Source: CAD feature listing. Evaluate the final solid. Frame: model axes, mm. A direction names the side the tool comes from. Give positions to 0.01 mm unless a question says otherwise; leave off trailing zeros. Loops run counter-clockwise (first coordinate to the right, second up) from the corner with the lowest first, then second, coordinate; pieces in that order, holes last. Notation, with made-up numbers: M 31,53.25 L 75,53.25 A21 cw 75,64.25 Z; hole C -6.5,0 d2. An arc over 180 degrees is marked long. Put each result on its own line as item: value.
from build123d import *

# Parameters (mm, degrees)
F0_R      = 37.95
F1_DEPTH  = 5
F2_R      = 36.45
F3_DEPTH  = 5
F4_R      = 3.25
F5_DEPTH  = 10
F6_R      = 12.5
F7_DEPTH  = 25
F8_R      = 9
F9_DEPTH  = 25
F10_R     = 1.5
F11_DEPTH = 10
F12_R     = 1.5
F13_DEPTH = 10


with BuildPart() as f1:
    # F0 (on Top) → F1 (new body)
    with BuildSketch(Plane.XY):
        Circle(F0_R)
    extrude(amount=F1_DEPTH)

    # F2 (on face) → F3 (join)
    with BuildSketch(Plane(origin=(0, 0, 0), x_dir=(1, 0, 0), z_dir=(0, 0, -1))):
        Circle(F2_R)
    extrude(amount=F3_DEPTH)

    # F4 (on face) → F5 (cut)
    with BuildSketch(Plane.XY.offset(5)):
        Circle(F4_R)
    extrude(amount=-F5_DEPTH, mode=Mode.SUBTRACT)

    # F6 (on face) → F7 (join)
    with BuildSketch(Plane.XY.offset(5)):
        with Locations((14.016853, 16.956646)):
            Circle(F6_R)
    extrude(amount=F7_DEPTH)

    # F8 (on face) → F9 (cut)
    with BuildSketch(Plane.XY.offset(30)):
        with Locations((14.016853, 16.956646)):
            Circle(F8_R)
    extrude(amount=-F9_DEPTH, mode=Mode.SUBTRACT)

    # F10 (on face) → F11 (cut)
    with BuildSketch(Plane.XY.offset(5)):
        with Locations((24.087269, -16.958203)):
            Circle(F10_R)
    extrude(amount=-F11_DEPTH, mode=Mode.SUBTRACT)

    # F12 (on Front) → F13 (cut)
    with BuildSketch(Plane.XZ):
        with Locations((12.184734, 11.070393)):
            Circle(F12_R)
    extrude(amount=-F13_DEPTH, mode=Mode.SUBTRACT)


solid = f1.part
1. Section query C-C (y = 18.5). Output: boundary loops of the cut face in (x, z).
Found:
outline: M -33.14,0 L -31.41,0 L -31.41,-5 L 31.41,-5 L 31.41,0 L 33.14,0 L 33.14,5 L 26.42,5 L 26.42,30 L 22.88,30 L 22.88,5 L 5.15,5 L 5.15,30 L 1.61,30 L 1.61,5 L -33.14,5 Z
2. Material intervals for line 1 (X direction, y = 17.5, z = 13); line 2 (Y direction, x = 0, z = 2); line 3 (Z direction, x = -2, y = 17.5), sorted ascending. Write a range as from..to.
Found:
line 1: 1.53..5.03, 23..26.51
line 2: -37.95..-3.25, 3.25..37.95
line 3: -5..5
3. Section query D-D (x = -26.5). Output: boundary loops of the cut face in (y, z), plus the area to 3 significant figures.
Found:
outline: M -27.17,0 L -25.03,0 L -25.03,-5 L 25.03,-5 L 25.03,0 L 27.17,0 L 27.17,5 L -27.17,5 Z
area: 522 mm^2
4. Access query for faces 1 (the flat face through (-34, 14, 0)), 2 (the cylindrical face through (25.52, -16.51, 0.07)), 3 (the cylindrical face through (18.855, 24.545, 17.675)). Directions: +Z, -Z, +X, -X, +Y, -Y. A direction counts if a zero-diameter tool reaches every point of the face in a straight line with its end or side. Return the directions, or none.
Found:
face 1: -Z
face 2: +Z, -Z
face 3: +Z
5. Contact query for flat-ended pins moving along their axis: P1, Ø4, axis at y = 25.5, z = 1.5, coming from the +X side; P2, Ø14.5, axis at x = 14.5, y = 15.5, coming from the +Z side; P3, Ø12, axis at x = 5, z = 19, coming from the -Y side; P4, Ø2.5, axis at x = 24.09, y = -16.96, coming from the -Z side. Output: stop coordinate, or through.
Found:
P1: x = 29.8
P2: z = 5
P3: y = 4.83
P4: through
6. Draft query along X for faces 4 (the cylindrical face through (11.86, 6.504, 9.606)), 5 (the cylindrical face through (20.737, 27.497, 17.325)), 6 (the flat face through (-1, -8, 5)). Return one class per face: pulls with the +X half, pulls with the -X half, needs draft (parallel to the pull), parting line crosses it, or undercut.
Found:
face 4: undercut
face 5: parting line crosses it
face 6: needs draft
7. Section query A-A (x = 0). Output: boundary loops of the cut face in (y, z), plus the area to 3 significant figures.
Found:
outline: M -37.95,0 L -36.45,0 L -36.45,-5 L -3.25,-5 L -3.25,5 L -37.95,5 Z; M 3.25,-5 L 36.45,-5 L 36.45,0 L 37.95,0 L 37.95,5 L 3.25,5 Z
area: 679 mm^2
